Input: part model. Units: mm. Frame: model coordinates. A direction names the side the tool comes from. Coordinates: 2 decimals unless noted, no trailing zeros. Write each loop counter-clockwise with the first axis right and the second up, starting at its lowest first coordinate (ties: lowest second). Pieces come first, ordered by that corner, then holes. Notation, with made-up numbers: M 82,86 L 139,86 A32 ccw 139,112 Z; hole C 53.5,2.25 d11. An arc over 180 degrees is marked long. Write each question's results on one line, items separated by ' | '. Start each with the question number.
1. Set-up query: faces 4 (the cylindrical face through (-0.54, -2.44, 0.14)), 5 (the cylindrical face through (3.233, -1.341, -10.246)). Return all of +Z, -Z, +X, -X, +Y, -Y with unobstructed straight access to the full face (end or side cutting, diameter ignored); none if empty.
2. Section query A-A, the plane x = 0. Output: boundary loops of the cut face in (y, z), and give its area (4 significant figures).
3. Section query C-C, the plane z = 1. Output: boundary loops of the cut face in (x, y).
4. First-contact query: pin 1 (4 mm diameter, centred on y = -2.5, z = 4, fed in from +X); pin 2 (3 mm diameter, centred on y = 0.5, z = 4.5, fed in from -X); pin 3 (2 mm diameter, centred on x = 2.5, z = 3.5, fed in from -Y). Flat tips, straight axial feed; report the tip coordinate or a pass-through.
5. Ray query, probe 1 along Z at (x, y) = (2.75, 0.25); probe 2 along Y at (x, z) = (0, 0.5); probe 3 along X at (y, z) = (1.5, 2.75). Return the intervals inside material, ascending.
6. Pull-direction query (Z, two-part tool) for faces 1 (the cylindrical face through (3.233, -1.341, 10.246)), 2 (the flat face through (2, -2, -10)), 3 (the flat face through (0, 0, -11)); classes: +Z half, -Z half, draft (parallel to the pull), parting line (faces both ways), or undercut.
```python
from build123d import *

# Parameters (mm, degrees)
SKETCH1_R           = 2.5
BOSS_EXTRUDE1_DEPTH = 10
SKETCH2_R           = 3.5
BOSS_EXTRUDE2_DEPTH = 1
CHAMFER1_SIZE       = 0.5


with BuildPart() as part:
    # Sketch1 → Boss-Extrude1 (new body, symmetric)
    with BuildSketch(Plane.XY):
        Circle(SKETCH1_R)
    extrude(amount=BOSS_EXTRUDE1_DEPTH, both=True)

    # Sketch2 → Boss-Extrude2 (add)
    with BuildSketch(Plane.XY.offset(10)):
        Circle(SKETCH2_R)
    boss_extrude2 = extrude(amount=BOSS_EXTRUDE2_DEPTH)

    # Mirror1: Boss-Extrude2 across plane
    add(boss_extrude2.mirror(Plane.XY))

    # Chamfer1
    chamfer1_edges = [part.edges().sort_by_distance(p)[0] for p in [
        (-3.5, 0, 11),
        (-3.5, 0, -11),
    ]]
    chamfer(chamfer1_edges, length=CHAMFER1_SIZE)


solid = part.part
```
Answer:
1) face 4: none | face 5: +Z, -Z
2) outline: M -3.5,-10.5 L -3,-11 L 3,-11 L 3.5,-10.5 L 3.5,-10 L 2.5,-10 L 2.5,10 L 3.5,10 L 3.5,10.5 L 3,11 L -3,11 L -3.5,10.5 L -3.5,10 L -2.5,10 L -2.5,-10 L -3.5,-10 Z | area: 113.5 mm^2
3) outline: C 0,0 d5
4) pin 1: x = 2.45 | pin 2: x = -2.5 | pin 3: y = -2
5) probe 1: -11 to -10, 10 to 11 | probe 2: -2.5 to 2.5 | probe 3: -2 to 2
6) face 1: draft | face 2: undercut | face 3: -Z half
